```python
from build123d import *

# Parameters (mm, degrees)
F1_DEPTH = 41.275
F2_DEPTH = 14.2875
F4_R     = 5.55625
F5_DEPTH = 38.1


with BuildPart() as f1:
    # F0 (on Top) → F1 (new body)
    with BuildSketch(Plane.XY):
        with BuildLine():
            ThreePointArc((-21.4376, -31.75), (10.3124, 0), (-21.4376, 31.75))
            ThreePointArc((-21.4376, 31.75), (-39.882683, 25.842628), (-51.46402, 10.31875))
            Line((-51.46402, 10.31875), (-39.310199, 10.31875))
            ThreePointArc((-39.310199, 10.31875), (-0.8001, 0), (-39.310199, -10.31875))
            Line((-39.310199, -10.31875), (-51.46402, -10.31875))
            ThreePointArc((-51.46402, -10.31875), (-39.882683, -25.842628), (-21.4376, -31.75))
        make_face()
    extrude(amount=F1_DEPTH)

    # F0 (on Top) → F2 (join)
    with BuildSketch(Plane.XY):
        with BuildLine():
            ThreePointArc((-21.4376, -31.75), (10.3124, 0), (-21.4376, 31.75))
            ThreePointArc((-21.4376, 31.75), (-39.882683, 25.842628), (-51.46402, 10.31875))
            Line((-51.46402, 10.31875), (-39.310199, 10.31875))
            ThreePointArc((-39.310199, 10.31875), (-0.8001, 0), (-39.310199, -10.31875))
            Line((-39.310199, -10.31875), (-51.46402, -10.31875))
            ThreePointArc((-51.46402, -10.31875), (-39.882683, -25.842628), (-21.4376, -31.75))
        make_face()
        with BuildLine():
            Line((37.2999, 31.75), (-21.4376, 31.75))
            ThreePointArc((-21.4376, 31.75), (10.3124, 0), (-21.4376, -31.75))
            Line((-21.4376, -31.75), (37.2999, -31.75))
            ThreePointArc((37.2999, -31.75), (48.52522, -27.10032), (53.1749, -15.875))
            Line((53.1749, -15.875), (53.1749, -10.31875))
            Line((53.1749, -10.31875), (32.5374, -10.31875))
            ThreePointArc((32.5374, -10.31875), (22.219841, 0.156758), (32.850879, 10.313987))
            Line((32.850879, 10.313987), (53.1749, 10.313987))
            Line((53.1749, 10.313987), (53.1749, 15.875))
            ThreePointArc((53.1749, 15.875), (48.52522, 27.10032), (37.2999, 31.75))
        make_face()
    extrude(amount=F2_DEPTH)

    # F4 (on offset) → F5 (cut)
    with BuildSketch(Plane.YZ.offset(25.4)):
        with Locations((0, 26.9875)):
            Circle(F4_R)
    extrude(amount=-F5_DEPTH, mode=Mode.SUBTRACT)


solid = f1.part
```
Model file for the job. Use its own axes, mm. A direction names the side the tool comes from. Give positions to 0.01 mm unless a question says otherwise; leave off trailing zeros. Write each loop counter-clockwise with the first axis right and the second up, starting at its lowest first coordinate (ties: lowest second). Pieces come first, ordered by that corner, then holes. Notation, with made-up numbers: M -19,38.5 L 13,38.5 A14 cw 13,62.5 Z; hole C 26,24.25 d1. An arc over 180 degrees is marked long. Use a Markdown table: item, result.
1) Pin check, flat tips, straight feed: pin 1 (3 mm diameter, centred on x = -34.5, z = 14, fed in from +Y); pin 2 (7 mm diameter, centred on x = 47, z = 4, fed in from -Y); pin 3 (13 mm diameter, centred on y = 0, z = 26.99, fed in from -X); pin 4 (8 mm diameter, centred on x = -11, y = -12, fed in from +Z). Stop position of each tip, or through.
Responses:
| item | result |
|---|---|
| pin 1 | stops at y = 29.57 |
| pin 2 | stops at y = -30.49 |
| pin 3 | stops at x = -1.85 |
| pin 4 | passes through |
2) Tool access for faces 4 (the flat face through (-45, 10.319, 20)), 5 (the flat face through (12, 0, 0)), 6 (the flat face through (43, -10.319, 7)): list every direction of +Z, -Z, +X, -X, +Y, -Y with a clear straight run to the whole face (end or side of a thin tool).
Responses:
| item | result |
|---|---|
| face 4 | +Z, -Z, -X |
| face 5 | -Z, +X, -X, +Y, -Y |
| face 6 | +Z, -Z, +X |
3) Cut at B-B (x = 39.5). List the corners of the cut face in (y, z), and give its area (3 significant figures).
Responses:
| item | result |
|---|---|
| outline | M -31.6,0 L -10.32,0 L -10.32,14.29 L -31.6,14.29 Z; M 10.31,0 L 31.6,0 L 31.6,14.29 L 10.31,14.29 Z |
| area | 608 mm2 |
4) Drill centre lines: line 1 (Z direction, x = 19, y = 17); line 2 (Z direction, x = 4.5, y = 0) (3 decimals); line 3 (Y direction, x = -17, z = 3.5). Where is each one in solid material? Low to high. Write a range as from..to.
Responses:
| item | result |
|---|---|
| line 1 | z = 0..14.29 |
| line 2 | z = 0..21.431, 32.544..41.275 |
| line 3 | y = -31.75..-20.15, 20.15..31.75 |
5) Pull direction X, two halves, no side cores. Call faces 1 (the cylindrical face through (-0.814, 0.756, 20.349)), 2 (the flat face through (53.175, 13, 7)), 3 (the flat face through (43, 10.314, 7)): +X half, -X half, draft (parallel to the pull), parting line (faces both ways), or undercut.
Responses:
| item | result |
|---|---|
| face 1 | undercut |
| face 2 | +X half |
| face 3 | draft |
6) Cut at A-A (y = 0). List the corners of the cut face in (x, z) (1 decimal), and give its area (3 significant figures).
Responses:
| item | result |
|---|---|
| outline | M -0.8,0 L 22.2,0 L 22.2,14.3 L 10.3,14.3 L 10.3,21.4 L -0.8,21.4 Z; M -0.8,32.5 L 10.3,32.5 L 10.3,41.3 L -0.8,41.3 Z |
| area | 505 mm2 |
